from build123d import *

# Parameters (mm, degrees)
SKETCH1_R           = 9.5
BOSS_EXTRUDE1_DEPTH = 5.8
SKETCH2_R           = 8.75
CUT_EXTRUDE1_DEPTH  = 5.8
SKETCH3_W           = 1
SKETCH3_H           = 1
BOSS_EXTRUDE2_DEPTH = 5.8


with BuildPart() as part:
    # Sketch1 → Boss-Extrude1 (new body)
    with BuildSketch(Plane.XY):
        with Locations((-43.212664647, 1.441865661)):
            Circle(SKETCH1_R)
    extrude(amount=BOSS_EXTRUDE1_DEPTH)

    # Sketch2 → Cut-Extrude1 (cut)
    with BuildSketch(Plane.XY.offset(5.8)):
        with Locations((-43.212664647, 1.441865661)):
            Circle(SKETCH2_R)
    extrude(amount=-CUT_EXTRUDE1_DEPTH, mode=Mode.SUBTRACT)

    # Sketch3 → Boss-Extrude2 (add)
    with BuildSketch(Plane.XY.offset(5.8)):
        Polygon((-40.889172194, 11.129687027), (-39.92967922, 10.84795447), (-40.211411777, 9.888461496), (-41.170904751, 10.170194053), align=None)
        with Locations((-43.212664647, 10.891865661)):
            Rectangle(SKETCH3_W, SKETCH3_H)
        Polygon((-38.25391528, 10.082658721), (-37.412661747, 9.542017904), (-37.953302565, 8.700764371), (-38.794556098, 9.241405188), align=None)
        Polygon((-36.02038675, 8.335604751), (-35.365526016, 7.579855176), (-36.12127559, 6.924994442), (-36.776136324, 7.680744017), align=None)
        Polygon((-34.3695338, 6.030061038), (-33.954118787, 5.120429043), (-34.863750783, 4.70501403), (-35.279165796, 5.614646025), align=None)
        Polygon((-33.43509872, 3.352809023), (-33.292783882, 2.362987581), (-34.282605324, 2.220672742), (-34.424920162, 3.210494184), align=None)
        Polygon((-33.292783882, 0.520743741), (-33.43509872, -0.469077701), (-34.424920162, -0.326762863), (-34.282605324, 0.663058579), align=None)
        Polygon((-33.954118787, -2.236697721), (-34.3695338, -3.146329716), (-35.279165796, -2.730914703), (-34.863750783, -1.821282708), align=None)
        Polygon((-35.365526016, -4.696123855), (-36.02038675, -5.451873429), (-36.776136324, -4.797012695), (-36.12127559, -4.041263121), align=None)
        Polygon((-37.412661747, -6.658286582), (-38.25391528, -7.1989274), (-38.794556098, -6.357673867), (-37.953302565, -5.817033049), align=None)
        Polygon((-39.92967922, -7.964223148), (-40.889172194, -8.245955705), (-41.170904751, -7.286462731), (-40.211411777, -7.004730175), align=None)
        with Locations((-43.212664647, -8.008134339)):
            Rectangle(SKETCH3_W, SKETCH3_H)
        Polygon((-45.536157101, -8.245955705), (-46.495650075, -7.964223148), (-46.213917518, -7.004730175), (-45.254424544, -7.286462731), align=None)
        Polygon((-48.171414015, -7.1989274), (-49.012667548, -6.658286582), (-48.47202673, -5.817033049), (-47.630773197, -6.357673867), align=None)
        Polygon((-50.404942545, -5.451873429), (-51.059803279, -4.696123855), (-50.304053705, -4.041263121), (-49.649192971, -4.797012695), align=None)
        Polygon((-52.055795495, -3.146329716), (-52.471210508, -2.236697721), (-51.561578512, -1.821282708), (-51.146163499, -2.730914703), align=None)
        Polygon((-52.990230575, -0.469077701), (-53.132545413, 0.520743741), (-52.142723971, 0.663058579), (-52.000409133, -0.326762863), align=None)
        Polygon((-53.132545413, 2.362987581), (-52.990230575, 3.352809023), (-52.000409133, 3.210494184), (-52.142723971, 2.220672742), align=None)
        Polygon((-52.471210508, 5.120429043), (-52.055795495, 6.030061038), (-51.146163499, 5.614646025), (-51.561578512, 4.70501403), align=None)
        Polygon((-51.059803279, 7.579855176), (-50.404942545, 8.335604751), (-49.649192971, 7.680744017), (-50.304053705, 6.924994442), align=None)
        Polygon((-49.012667548, 9.542017904), (-48.171414015, 10.082658721), (-47.630773197, 9.241405188), (-48.47202673, 8.700764371), align=None)
        Polygon((-46.495650075, 10.84795447), (-45.536157101, 11.129687027), (-45.254424544, 10.170194053), (-46.213917518, 9.888461496), align=None)
    extrude(amount=-BOSS_EXTRUDE2_DEPTH)


solid = part.part
Input: part model. Units: mm. Frame: model coordinates. A direction names the side the tool comes from. Give positions to 0.01 mm unless a question says otherwise; leave off trailing zeros. Order: outer loops, then holes, each group sorted by start corner. A loop starts at its lowest first (then second) coordinate and runs counter-clockwise, first axis right, second up.
Q1. Draft query along Y for faces 1 (the cylindrical face through (-34.1, -1.25, 2.86)), 2 (the flat face through (-40.42, 10.99, 2.94)), 3 (the flat face through (-33.363, 0.033, 2.941)), 4 (the cylindrical face through (-36.98, 8.61, 2.86)). Return one class per face: +Y half, -Y half, draft (parallel to the pull), parting line (faces both ways), or undercut.
Checked values:
face 1: undercut
face 2: +Y half
face 3: -Y half
face 4: undercut
Q2. Ray query, probe 1 along Y at (x, z) = (-37.5, 2.15); probe 2 along Y at (x, z) = (-43, 2.8); probe 3 along X at (y, z) = (-1.25, 4.75). Return the intervals inside material, ascending.
Checked values:
probe 1: y = -6.71 to -6.52, -6.15 to -5.19, 8.07 to 9.03, 9.41 to 9.6
probe 2: y = -8.51 to -7.31, 10.19 to 11.39
probe 3: x = -52.32 to -51.54, -34.89 to -34.1
Q3. Section B-B on y = -1.25. Output: boundary loops of the cut face in (x, z), and give its area (3 significant figures).
Checked values:
outline: (-52.32, 0) - (-51.54, 0) - (-51.54, 5.8) - (-52.32, 5.8) - close; (-34.89, 0) - (-34.1, 0) - (-34.1, 5.8) - (-34.89, 5.8) - close
area: 9.11 mm2
Q4. Contact query for flat-ended pins moving along their axis: pin 1 Ø10 at (x, y) = (-45, -2) entering from +Z; pin 2 Ø3 at (y, z) = (-1.5, 4.5) entering from -X; pin 3 Ø3 at (x, z) = (-46.5, 2) entering from +Y; pin 4 Ø3 at (x, z) = (-51, 1.5) entering from +Y. Output: stop coordinate, or through.
Checked values:
pin 1: stops at z = 5.8
pin 2: stops at x = -53.06
pin 3: stops at y = 11.13
pin 4: stops at y = 8.56
Q5. Section A-A on x = -48.5. Output: boundary loops of the cut face in (y, z).
Checked values:
outline: (-6.99, 0) - (-5.53, 0) - (-5.53, 5.8) - (-6.99, 5.8) - close; (8.41, 0) - (9.87, 0) - (9.87, 5.8) - (8.41, 5.8) - close
Q6. Set-up query: faces 5 (the flat face through (-46.023, 10.987, 2.941)), 6 (the cylindrical face through (-37.001, -5.746, 2.859)), 7 (the cylindrical face through (-41.873, -7.963, 2.859)). Return all of +Z, -Z, +X, -X, +Y, -Y with unobstructed straight access to the full face (end or side cutting, diameter ignored); none if empty.
Checked values:
face 5: +Z, -Z, -X, +Y
face 6: +Z, -Z
face 7: +Z, -Z, -Y
